Autodesk Inventor part; units mm, degrees
ref_plane "YZ Plane" through (0, 0, 0) normal (1, 0, 0) x (0, 1, 0)
ref_plane "XZ Plane" through (0, 0, 0) normal (0, 1, 0) x (-1, 0, 0)
ref_plane "XY Plane" through (0, 0, 0) normal (0, 0, 1) x (1, 0, 0)
sketch "Esboço1" plane through (0, 0, 0) normal (0, 1, 0) x (-1, 0, 0)
  line L0 (-5, 101.6) -> (5, 101.6)
  line L1 (5, 101.6) -> (5, -101.6)
  line L2 (5, -101.6) -> (-5, -101.6)
  line L3 (-5, -101.6) -> (-5, 101.6)
  line L4 (-5, 101.6) -> (5, -101.6) construction
  line L5 (5, 101.6) -> (-5, -101.6) construction
  point P0 (0, 0)
  dimension "d0" = 203.2
  dimension "d1" = 10
extrude "Extrusão1" add sketch "Esboço1" along normal blind 30
sketch "Esboço3" plane through (5, 0, 101.6) normal (1, 0, 0) x (0, 0, -1)
  line L0 (203.2, 30) -> (0, 30)
  circle A0 centre (101.6, 15) radius 12.5
  line L1 (0, 0) -> (203.2, 0)
  line L2 (203.2, 0) -> (203.2, 30)
  line L3 (203.2, 0) -> (0, 0)
  point P0 (101.6, 0)
  point P1 (101.6, 0)
  point P2 (101.6, 0)
  dimension "d4" = 25
  dimension "d7" = 15
  dimension "d10" = 0
extrude "Extrusão2" cut sketch "Esboço3" against normal blind 30
properties part number "exHelice"
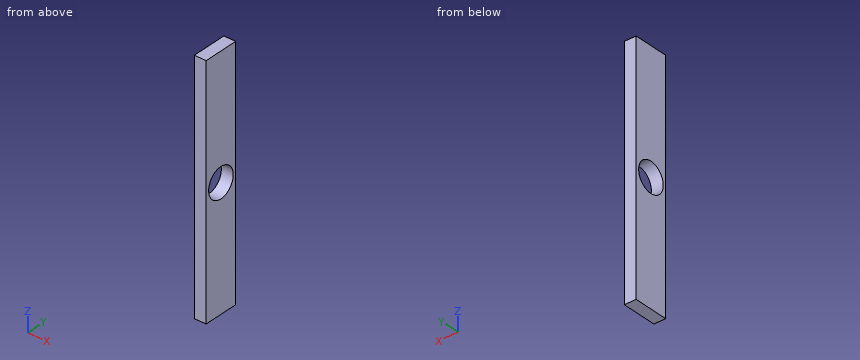
Build history of the part. All positions in model axes, mm. Give positions to 0.01 mm unless a question says otherwise; leave off trailing zeros. Loops run counter-clockwise (first coordinate to the right, second up) from the corner with the lowest first, then second, coordinate; pieces in that order, holes last.
Item 1: Slice it at B-B, the plane y = 15. List the corners of the cut face in (x, z), and give its area (3 significant figures).
Answers follow:
outline: (-5, -101.6) - (5, -101.6) - (5, -12.5) - (-5, -12.5) - close; (-5, 12.5) - (5, 12.5) - (5, 101.6) - (-5, 101.6) - close
area: 1,780 mm2
Item 2: Slice it at A-A, the plane z = 0. List the corners of the cut face in (x, y).
Answers follow:
outline: (-5, 0) - (5, 0) - (5, 2.5) - (-5, 2.5) - close; (-5, 27.5) - (5, 27.5) - (5, 30) - (-5, 30) - close
Item 3: Drill centre lines: line 1 (Y direction, x = 0, z = 0); line 2 (Z direction, x = -4, y = 9.5); line 3 (Z direction, x = 1.25, y = 18). Where is each one in solid material? Low to high.
Answers follow:
line 1: y = 0 to 2.5, 27.5 to 30
line 2: z = -101.6 to -11.22, 11.22 to 101.6
line 3: z = -101.6 to -12.13, 12.13 to 101.6
Item 4: Slice it at C-C, the plane x = 0.25. List the corners of the cut face in (y, z).
Answers follow:
outline: (0, -101.6) - (30, -101.6) - (30, 101.6) - (0, 101.6) - close; hole circle Ø25 at (15, 0)
Item 5: Flat gauge pin, fed straight in: pin 1 (4 mm diameter, centred on x = -3.5, z = 21.5, fed in from -Y). Where does the tip first touch, or does it go through?
Answers follow:
pin 1: stops at y = 0
